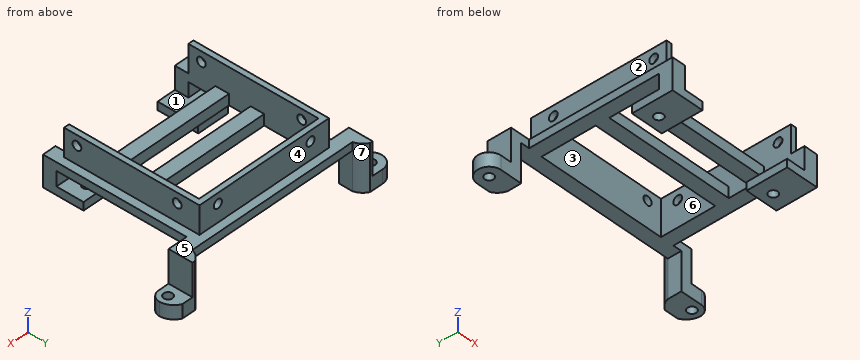
from build123d import *

# Parameters (mm, degrees)
CROQUIS1_R                = 1.625
SALIENTE_EXTRUIR1_DEPTH   = 5
SALIENTE_EXTRUIR1_2_DEPTH = 5
SALIENTE_EXTRUIR2_DEPTH   = 12
SALIENTE_EXTRUIR4_DEPTH   = 3
SALIENTE_EXTRUIR6_DEPTH   = 10.25
CROQUIS12_R               = 1.625
CORTAR_EXTRUIR1_DEPTH     = 51.7
CROQUIS13_R               = 1.625
CORTAR_EXTRUIR2_DEPTH     = 2
CROQUIS14_W               = 5
CROQUIS14_H               = 5
SALIENTE_EXTRUIR7_DEPTH   = 11.4
CROQUIS15_W               = 11.9
CROQUIS15_H               = 14.969217292
CROQUIS15_R               = 1.625
SALIENTE_EXTRUIR8_DEPTH   = 3
CROQUIS16_W               = 47.7
CROQUIS16_H               = 5
SALIENTE_EXTRUIR9_DEPTH   = 4


with BuildPart() as part:
    # Croquis1 → Saliente-Extruir1 (new body)
    with BuildSketch(Plane.XY):
        with BuildLine():
            Line((190, -61.4), (182, -61.4))
            Line((182, -61.4), (182, -56.4))
            ThreePointArc((182, -56.4), (183.099702641, -54.183975769), (185, -52.6))
            Line((185, -52.6), (190, -52.6))
            ThreePointArc((190, -52.6), (192.511852896, -54.746889597), (193.5, -57.9))
            ThreePointArc((193.5, -57.9), (192.474873734, -60.374873734), (190, -61.4))
        make_face()
        with Locations((190, -57.9)):
            Circle(CROQUIS1_R, mode=Mode.SUBTRACT)
    extrude(amount=SALIENTE_EXTRUIR1_DEPTH)



with BuildPart() as body_2:
    # Croquis1 → Saliente-Extruir1 2 (new body)
    with BuildSketch(Plane.XY):
        with BuildLine():
            Line((115, -52.6), (110, -52.6))
            ThreePointArc((110, -52.6), (105.6, -57), (110, -61.4))
            Line((110, -61.4), (118, -61.4))
            Line((118, -61.4), (118, -56.4))
            ThreePointArc((118, -56.4), (116.900297359, -54.183975769), (115, -52.6))
        make_face()
        with Locations((110, -57)):
            Circle(CROQUIS1_R, mode=Mode.SUBTRACT)
    extrude(amount=SALIENTE_EXTRUIR1_2_DEPTH)


with BuildPart() as part_1:
    add(part.part)

    add(body_2.part)  # Saliente-Extruir2 merges body 2
    # Croquis4 → Saliente-Extruir2 (add)
    with BuildSketch(Plane.XY.offset(5)):
        with BuildLine():
            Line((115, -52.6), (114, -52.6))
            Line((114, -52.6), (114, -61.4))
            Line((114, -61.4), (118, -61.4))
            Line((118, -61.4), (118, -56.4))
            ThreePointArc((118, -56.4), (116.900297359, -54.183975769), (115, -52.6))
        make_face()
        with BuildLine():
            Line((185, -52.6), (186, -52.6))
            Line((186, -52.6), (186, -61.4))
            Line((186, -61.4), (182, -61.4))
            Line((182, -61.4), (182, -56.4))
            ThreePointArc((182, -56.4), (183.099702641, -54.183975769), (185, -52.6))
        make_face()
    extrude(amount=SALIENTE_EXTRUIR2_DEPTH)

    # Croquis7 → Saliente-Extruir4 (add)
    with BuildSketch(Plane.XY.offset(17)):
        Polygon((118, -56.4), (182, -56.4), (182, -61.4), (178.85, -61.4), (178.85, -109.35), (173.85, -109.35), (173.85, -61.4), (170.85, -61.4), (129.15, -61.4), (126.15, -61.4), (126.15, -109.35), (121.15, -109.35), (121.15, -61.4), (118, -61.4), align=None)
    extrude(amount=-SALIENTE_EXTRUIR4_DEPTH)

    # Croquis10 → Saliente-Extruir6 (add)
    with BuildSketch(Plane.XY.offset(17)):
        Polygon((124.15, -59.4), (126.15, -59.4), (173.85, -59.4), (175.85, -59.4), (175.85, -109.35), (173.85, -109.35), (173.85, -61.4), (126.15, -61.4), (126.15, -109.35), (124.15, -109.35), align=None)
    extrude(amount=SALIENTE_EXTRUIR6_DEPTH)

    # Croquis12 → Cortar-Extruir1 (cut)
    with BuildSketch(Plane.ZY.offset(-124.15)):
        with Locations((23.5, -67.6)):
            Circle(CROQUIS12_R)
        with Locations((23.5, -104.6)):
            Circle(CROQUIS12_R)
    extrude(amount=-CORTAR_EXTRUIR1_DEPTH, mode=Mode.SUBTRACT)

    # Croquis13 → Cortar-Extruir2 (cut)
    with BuildSketch(Plane(origin=(0, -59.4, 0), x_dir=(1, 0, 0), z_dir=(0, 1, 0))):
        with Locations(Location((131.5, -23.5, 0), (0, 0, 270))):
            Circle(CROQUIS13_R)
        with Locations(Location((168.5, -23.5, 0), (0, 0, 270))):
            Circle(CROQUIS13_R)
    extrude(amount=-CORTAR_EXTRUIR2_DEPTH, mode=Mode.SUBTRACT)

    # Croquis14 → Saliente-Extruir7 (add)
    with BuildSketch(Plane.XY.offset(17)):
        with Locations((123.65, -111.85)):
            Rectangle(CROQUIS14_W, CROQUIS14_H)
        with Locations((176.35, -111.85)):
            Rectangle(CROQUIS14_W, CROQUIS14_H)
    extrude(amount=-SALIENTE_EXTRUIR7_DEPTH)

    # Croquis15 → Saliente-Extruir8 (add)
    # profile 1 of 2: a face of its own
    with BuildSketch(Plane(origin=(0, 0, 5.6), x_dir=(-1, 0, 0), z_dir=(0, 0, -1))):
        with Locations((-172.9, -106.865391354)):
            Rectangle(CROQUIS15_W, CROQUIS15_H)
        with Locations((-172.9, -103.7)):
            Circle(CROQUIS15_R, mode=Mode.SUBTRACT)
    # profile 2 of 2: a face of its own
    with BuildSketch(Plane(origin=(0, 0, 5.6), x_dir=(-1, 0, 0), z_dir=(0, 0, -1))):
        with Locations((-127.1, -106.865391354)):
            Rectangle(CROQUIS15_W, CROQUIS15_H)
        with Locations((-127.1, -103.8)):
            Circle(CROQUIS15_R, mode=Mode.SUBTRACT)
    extrude(amount=-SALIENTE_EXTRUIR8_DEPTH)

    # Croquis16 → Saliente-Extruir9 (add)
    with BuildSketch(Plane(origin=(0, 0, 14), x_dir=(-1, 0, 0), z_dir=(0, 0, -1))):
        with Locations((-150, -83.9)):
            Rectangle(CROQUIS16_W, CROQUIS16_H)
        with Locations((-150, -96.9)):
            Rectangle(CROQUIS16_W, CROQUIS16_H)
    extrude(amount=-SALIENTE_EXTRUIR9_DEPTH)


solid = part_1.part
For this review, take the finished solid that the model builds, in its own axes (mm). Face numbers are marked on the shaded views. A direction names the side the tool comes from. Round coordinates to 2 decimals unless told otherwise and drop trailing zeros. Write each loop counter-clockwise with the first axis right and the second up, starting at its lowest first coordinate (ties: lowest second). Pieces come first, ordered by that corner, then holes. Notation, with made-up numbers: (28.5, 30.5) - (74.5, 30.5) arc R19 ccw to (74.5, 59.5) - close; hole circle Ø7 at (50, -28). An arc over 180 degrees is marked (long way). Use a Markdown table: item, result.
Q1. We need section C-C (y = -67.6). Give the boundary of the cut face in (x, z) (3 decimals).
Derived:
| item | result |
|---|---|
| outline | (121.15, 14) - (126.15, 14) - (126.15, 21.875) - (124.15, 21.875) - (124.15, 17) - (121.15, 17) - close; (124.15, 25.125) - (126.15, 25.125) - (126.15, 27.25) - (124.15, 27.25) - close; (173.85, 14) - (178.85, 14) - (178.85, 17) - (175.85, 17) - (175.85, 21.875) - (173.85, 21.875) - close; (173.85, 25.125) - (175.85, 25.125) - (175.85, 27.25) - (173.85, 27.25) - close |
Q2. We need section B-B (x = 136.5). Give the boundary of the cut face in (y, z).
Derived:
| item | result |
|---|---|
| outline | (-99.4, 14) - (-94.4, 14) - (-94.4, 18) - (-99.4, 18) - close; (-86.4, 14) - (-81.4, 14) - (-81.4, 18) - (-86.4, 18) - close; (-61.4, 14) - (-56.4, 14) - (-56.4, 17) - (-59.4, 17) - (-59.4, 27.25) - (-61.4, 27.25) - close |
Q3. Machinability: for the marked faces 1, 2, 3 and 4, which of the approach directions +Z, -Z, +X, -X, +Y, -Y give a long, thin tool a straight path to every point of the face, cutting with its end or side? Answer none if there is none.
Derived:
| item | result |
|---|---|
| face 1 | +Y |
| face 2 | +Z, -X, +Y, -Y |
| face 3 | +Z, -Z |
| face 4 | +Z, +X, -X, +Y |
Q4. Wall thickness on line 1 along X through (y, z) = (-59.8, 23.5) (3 decimals); line 2 along Y through (x, z) = (125, 23.5) (3 decimals); line 3 along Y through (x, z) = (169.5, 17.25): over which ranges is each line inside the solid? List them lowest first.
Derived:
| item | result |
|---|---|
| line 1 | x = 124.15 to 129.875, 133.125 to 166.875, 170.125 to 175.85 |
| line 2 | y = -109.35 to -106.225, -102.975 to -69.225, -65.975 to -59.4 |
| line 3 | y = -99.4 to -94.4, -86.4 to -81.4, -61.4 to -59.4 |
Q5. We need section A-A (z = 10.25). Give the boundary of the cut face in (x, y), plus the area to 3 significant figures.
Derived:
| item | result |
|---|---|
| outline | (114, -61.4) - (118, -61.4) - (118, -56.4) arc R6 ccw to (115, -52.6) - (114, -52.6) - close; (121.15, -114.35) - (126.15, -114.35) - (126.15, -109.35) - (121.15, -109.35) - close; (173.85, -114.35) - (178.85, -114.35) - (178.85, -109.35) - (173.85, -109.35) - close; (182, -61.4) - (186, -61.4) - (186, -52.6) - (185, -52.6) arc R6 ccw to (182, -56.4) - close |
| area | 112 mm2 |
Q6. Clearance check with flat-ended pins moving along their axes: pin 1 (3 mm diameter, centred on y = -74.5, z = 23.5, fed in from +X); pin 2 (3.5 mm diameter, centred on y = -94, z = 13.5, fed in from -X); pin 3 (5.5 mm diameter, centred on x = 115, z = 10, fed in from -Y). State where each tip first meets the part, or that it passes through.
Derived:
| item | result |
|---|---|
| pin 1 | stops at x = 175.85 |
| pin 2 | stops at x = 121.15 |
| pin 3 | stops at y = -61.4 |
Q7. We need section D-D (x = 168.5). Give the boundary of the cut face in (y, z) (3 decimals), plus the area to 3 significant figures.
Derived:
| item | result |
|---|---|
| outline | (-114.35, 5.6) - (-99.381, 5.6) - (-99.381, 8.6) - (-114.35, 8.6) - close; (-99.4, 14) - (-94.4, 14) - (-94.4, 18) - (-99.4, 18) - close; (-86.4, 14) - (-81.4, 14) - (-81.4, 18) - (-86.4, 18) - close; (-61.4, 14) - (-56.4, 14) - (-56.4, 17) - (-59.4, 17) - (-59.4, 21.875) - (-61.4, 21.875) - close; (-61.4, 25.125) - (-59.4, 25.125) - (-59.4, 27.25) - (-61.4, 27.25) - close |
| area | 114 mm2 |
Q8. The part is to be moulded in two halves that separate along Y. For the marked faces 5, 6 and 7, say which applies: pulls with the +Y half, pulls with the -Y half, needs draft (parallel to the pull), parting line crosses it, or undercut.
Derived:
| item | result |
|---|---|
| face 5 | needs draft |
| face 6 | undercut |
| face 7 | pulls with the +Y half |
